Design review of the part built by this model. Coordinates are the model's own, in mm. Face numbers are marked on the shaded views. Give positions to 0.01 mm unless a question says otherwise; leave off trailing zeros. Write each loop counter-clockwise with the first axis right and the second up, starting at its lowest first coordinate (ties: lowest second). Pieces come first, ordered by that corner, then holes. Notation, with made-up numbers: M 49.5,-14.75 L 88.5,-14.75 A6 cw 88.5,-3.75 Z; hole C 54.5,35.5 d5. An arc over 180 degrees is marked long. One line per item, written item: value. Start each with the question number.
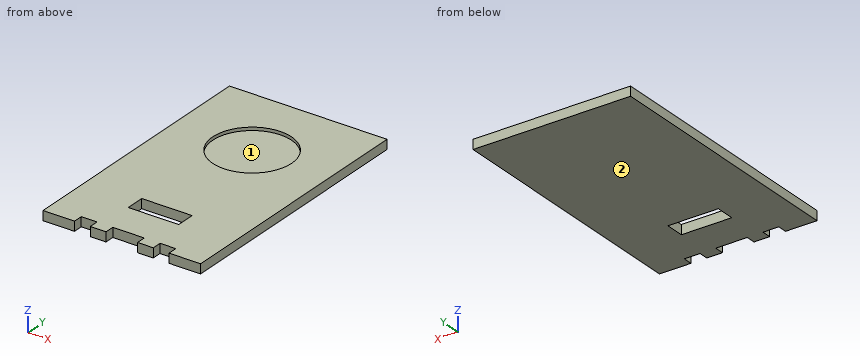
```python
from build123d import *

# Parameters (mm, degrees)
SKETCH1_W            = 16
SKETCH1_H            = 6
BOSS_EXTRUDE1_DEPTH  = 3
MOVE_FACE1_OUTLINE_W = 5
MOVE_FACE1_OUTLINE_H = 53.1
MOVE_FACE1_DEPTH     = 3
MOVE_FACE2_BY        = 30
SKETCH2_R            = 12.5
CUT_EXTRUDE1_DEPTH   = 1


# Read off the part's stored shape, not the designer's step: Move Face1
with BuildPart() as part:
    # Sketch1 → Boss-Extrude1 (new body)
    with BuildSketch(Plane.XY):
        Polygon((-20, 20), (-20, -30.1), (-20, -33.1), (-15, -33.1), (-15, -30.1), (-10, -30.1), (-10, -33.1), (-5, -33.1), (-5, -30.1), (5, -30.1), (5, -33.1), (10, -33.1), (10, -30.1), (15, -30.1), (15, -33.1), (20, -33.1), (20, -30.1), (20, 20), align=None)
        with Locations((0, -16)):
            Rectangle(SKETCH1_W, SKETCH1_H, mode=Mode.SUBTRACT)
    extrude(amount=BOSS_EXTRUDE1_DEPTH)

    # Move Face1 outline → Move Face1 (add)
    with BuildSketch(Plane.XY):
        with Locations((22.5, -6.55)):
            Rectangle(MOVE_FACE1_OUTLINE_W, MOVE_FACE1_OUTLINE_H)
        with Locations((-22.5, -6.55)):
            Rectangle(MOVE_FACE1_OUTLINE_W, MOVE_FACE1_OUTLINE_H)
    extrude(amount=MOVE_FACE1_DEPTH)

    # Move Face2: a face moved outward by 30.0
    extrude(part.faces().sort_by_distance((0, 20, 1.5))[0], amount=MOVE_FACE2_BY, dir=(0, 1, 0))

    # Sketch2 → Cut-Extrude1 (cut)
    with BuildSketch(Plane.XY.offset(3)):
        with Locations((0, 25)):
            Circle(SKETCH2_R)
    extrude(amount=-CUT_EXTRUDE1_DEPTH, mode=Mode.SUBTRACT)


solid = part.part
```
Q1. Wall thickness on line 1 (Y direction, x = 0, z = 2.4); line 2 (Y direction, x = 1.5, z = 1.65); line 3 (Y direction, x = -11.5, z = 2.5): over which ranges is each line inside the solid? List them lowest first. Write a range as from..to.
Q2. Take a section at C-C, the plane y = 25. Give the boundary of the cut face in (x, z), then the cut area to 3 significant figures.
Q3. Take a section at B-B, the plane x = 0. Give the boundary of the cut face in (y, z).
Q4. For P1, Ø0.9, axis at x = -1, z = 2, coming from the -Y side; P2, Ø20, axis at x = -1.5, y = 19.5, coming from the +Z side, all flat-tipped, find the tip position at first contact; note any pin that passes through.
Q5. The part is to be moulded in two halves that separate along X. For the marked faces 1 and 2, say which applies: pulls with the +X half, pulls with the -X half, needs draft (parallel to the pull), parting line crosses it, or undercut.
Q6. Take a section at D-D, the plane y = 33.5. Give the boundary of the cut face in (x, z).
Q7. Take a section at A-A, the plane z = 1. Give the boundary of the cut face in (x, y).
Results list:
1. line 1: y = -30.1..-19, -13..12.5, 37.5..50
1. line 2: y = -30.1..-19, -13..50
1. line 3: y = -30.1..20.1, 29.9..50
2. outline: M -25,0 L 25,0 L 25,3 L 12.5,3 L 12.5,2 L -12.5,2 L -12.5,3 L -25,3 Z
2. area: 125 mm^2
3. outline: M -30.1,0 L -19,0 L -19,3 L -30.1,3 Z; M -13,0 L 50,0 L 50,3 L 37.5,3 L 37.5,2 L 12.5,2 L 12.5,3 L -13,3 Z
4. P1: stops at y = -30.1
4. P2: stops at z = 3
5. face 1: undercut
5. face 2: needs draft
6. outline: M -25,0 L 25,0 L 25,3 L 9.17,3 L 9.17,2 L -9.17,2 L -9.17,3 L -25,3 Z
7. outline: M -25,-33.1 L -15,-33.1 L -15,-30.1 L -10,-30.1 L -10,-33.1 L -5,-33.1 L -5,-30.1 L 5,-30.1 L 5,-33.1 L 10,-33.1 L 10,-30.1 L 15,-30.1 L 15,-33.1 L 25,-33.1 L 25,50 L -25,50 Z; hole M -8,-19 L 8,-19 L 8,-13 L -8,-13 Z
